Autodesk Inventor part; units mm, degrees
ref_plane "YZ Plane" through (0, 0, 0) normal (1, 0, 0) x (0, 1, 0)
ref_plane "XZ Plane" through (0, 0, 0) normal (0, 1, 0) x (-1, 0, 0)
ref_plane "XY Plane" through (0, 0, 0) normal (0, 0, 1) x (1, 0, 0)
sketch "Sketch1" plane through (0, 0, 0) normal (0, 0, 1) x (1, 0, 0)
  line L0 (-64, -30) -> (64, -30)
  line L1 (64, -30) -> (64, 30)
  line L2 (64, 30) -> (-64, 30)
  line L3 (-64, 30) -> (-64, -30)
  line L4 (-64, -30) -> (64, 30) construction
  line L5 (64, -30) -> (-64, 30) construction
  point P0 (0, 0)
  dimension "d0" = 128
  dimension "d1" = 60
extrude "Extrusion1" add sketch "Sketch1" along normal blind 8
sketch "Sketch2" plane through (-64, 30, 0) normal (0, 1, 0) x (1, 0, 0)
  line L0 (128, 0) -> (0, 0)
  line L1 (0, 0) -> (0, -8)
  line L2 (128, -8) -> (0, -8)
  line L3 (128, 0) -> (128, -8)
  point P0 (64, 0)
  point P1 (5, -4)
  point P2 (123, -4)
  point P3 (64, -4)
  dimension "d4" = 5
  dimension "d5" = 5
hole "Hole1" at (-59, 30, 4) at (59, 30, 4) at (0, 30, 4) direction (0, -1, 0) diameter 5 end through all
sketch "Sketch3" plane through (-64, -30, 0) normal (0, -1, 0) x (1, 0, 0)
  point P0 (64, 0)
sketch "Sketch4" plane through (0, 0, 0) normal (0, 0, -1) x (-1, 0, 0)
  line L0 (0, 0) -> (0, 24.6794) construction
  point P0 (-28.0484, 0)
  point P1 (28.0484, 0)
hole "Hole2" at (-28.0484, 0, 0) at (28.0484, 0, 0) direction (0, 0, 1) diameter 48 end through all
properties part number "Separator1"
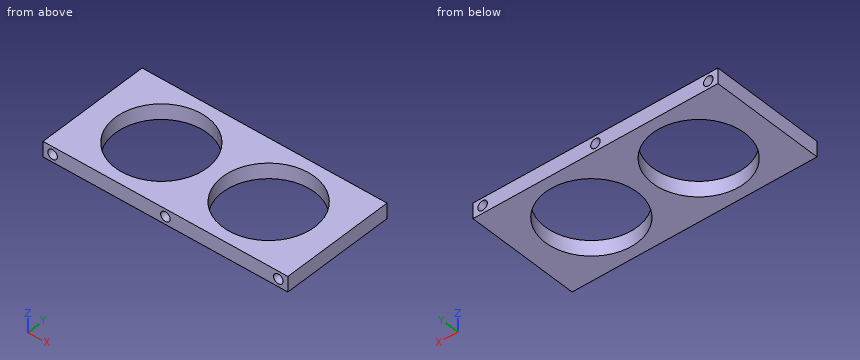
Can you work these out from the model? Positions are in its coordinate system, mm. Coordinates: 2 decimals unless noted, no trailing zeros. Write each loop counter-clockwise with the first axis right and the second up, starting at its lowest first coordinate (ties: lowest second). Pieces come first, ordered by that corner, then holes. Notation, with made-up numbers: (25.25, -29) - (56.25, -29) arc R19 ccw to (56.25, -8) - close; hole circle Ø7 at (-9.75, 51). An arc over 180 degrees is marked (long way). Return JSON: item names as keys, results as strings.
Q1. If we section it at D-D (y = -17): Please give me the cut outline in (x, z), then the cut area to 3 significant figures.
Computed values:
{"outline": "(-64, 0) - (-44.99, 0) - (-44.99, 8) - (-64, 8) - close; (-11.11, 0) - (11.11, 0) - (11.11, 8) - (-11.11, 8) - close; (44.99, 0) - (64, 0) - (64, 8) - (44.99, 8) - close; hole circle Ø5 at (-59, 4); hole circle Ø5 at (0, 4); hole circle Ø5 at (59, 4)", "area": "423 mm2"}
Q2. Please list where these lines run through material, in increasing order: L1, parallel to X at y = -10, z = 4.25; L2, parallel to X at y = 0, z = 2; L3, parallel to Z at x = 59, y = -13. Write a range as from..to.
Computed values:
{"L1": "x = -64..-61.49, -56.51..-49.87, -6.23..-2.49, 2.49..6.23, 49.87..56.51, 61.49..64", "L2": "x = -64..-60.5, -57.5..-52.05, -4.05..-1.5, 1.5..4.05, 52.05..57.5, 60.5..64", "L3": "z = 0..1.5, 6.5..8"}
Q3. If we section it at A-A (y = 0): Please give me the cut outline in (x, z), then the cut area to 3 significant figures.
Computed values:
{"outline": "(-64, 0) - (-52.05, 0) - (-52.05, 8) - (-64, 8) - close; (-4.05, 0) - (4.05, 0) - (4.05, 8) - (-4.05, 8) - close; (52.05, 0) - (64, 0) - (64, 8) - (52.05, 8) - close; hole circle Ø5 at (-59, 4); hole circle Ø5 at (0, 4); hole circle Ø5 at (59, 4)", "area": "197 mm2"}
Q4. If we section it at B-B (x = 0): Please give me the cut outline in (y, z), then the cut area to 3 significant figures.
Computed values:
{"outline": "(-30, 0) - (30, 0) - (30, 1.5) - (-30, 1.5) - close; (-30, 6.5) - (30, 6.5) - (30, 8) - (-30, 8) - close", "area": "180 mm2"}
Q5. If we section it at C-C (z = 3.5): Please give me the cut outline in (x, y).
Computed values:
{"outline": "(-64, -30) - (-61.45, -30) - (-61.45, 30) - (-64, 30) - close; (-56.55, -30) - (-2.45, -30) - (-2.45, 30) - (-56.55, 30) - close; (2.45, -30) - (56.55, -30) - (56.55, 30) - (2.45, 30) - close; (61.45, -30) - (64, -30) - (64, 30) - (61.45, 30) - close; hole circle Ø48 at (-28.05, 0); hole circle Ø48 at (28.05, 0)"}
